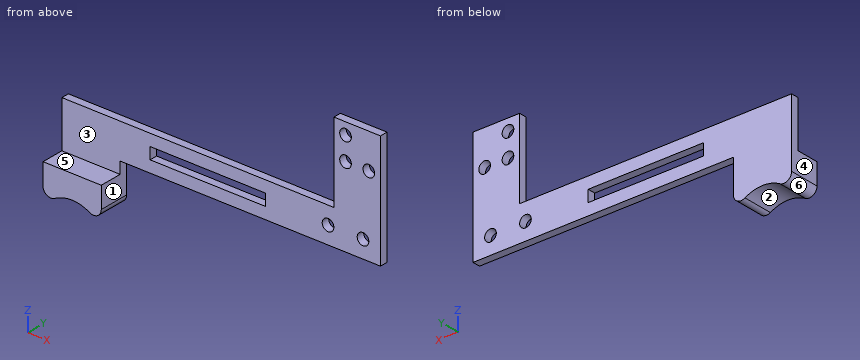
from build123d import *

# Parameters (mm, degrees)
F0_W      = 12
F0_H      = 16.5
F0_R      = 1.5
F0_W_2    = 15
F0_H_2    = 3
F1_DEPTH  = 2
F2_W      = 15
F2_H      = 7.8090135939
F3_DEPTH  = 10
F5_DEPTH  = 25
F6_R      = 2
F7_W      = 29.6666743584
F7_H      = 3
F8_DEPTH  = 25
F9_R      = 1.5
F10_DEPTH = 25


with BuildPart() as f1:
    # F0 (on Front) → F1 (new body)
    with BuildSketch(Plane.XZ):
        with Locations((3, -5.25)):
            Rectangle(F0_W, F0_H)
        with Locations((0, -6)):
            Circle(F0_R, mode=Mode.SUBTRACT)
        with Locations((6, -6)):
            Circle(F0_R, mode=Mode.SUBTRACT)
        Circle(F0_R, mode=Mode.SUBTRACT)
        Polygon((9, -13.5), (-3, -13.5), (-3, -17.375), (-3, -26.375), (9, -26.375), align=None)
        Polygon((-3, -26.375), (-3, -17.375), (-73, -17.375), (-73, -26.375), (-58, -26.375), align=None)
        with Locations((-65.5, -27.875)):
            Rectangle(F0_W_2, F0_H_2)
    extrude(amount=F1_DEPTH)

    # F2 (on face) → F3 (join)
    with BuildSketch(Plane(origin=(0, 0, -29.375), x_dir=(1, 0, 0), z_dir=(0, 0, -1))):
        with Locations((-65.5, 3.904506797)):
            Rectangle(F2_W, F2_H)
    extrude(amount=F3_DEPTH)

    # F4 (on face) → F5 (cut)
    with BuildSketch(Plane.XZ.offset(7.8090135939)):
        with BuildLine():
            Line((-73, -39.375), (-58, -39.375))
            ThreePointArc((-58, -39.375), (-65.5, -35.3883488839), (-73, -39.375))
        make_face()
    extrude(amount=-F5_DEPTH, mode=Mode.SUBTRACT)

    # F6
    f6_edges = [f1.edges().sort_by_distance(p)[0] for p in [
        (-73, -3.904507, -39.375),
        (-58, -3.904507, -39.375),
    ]]
    fillet(f6_edges, radius=F6_R)

    # F7 (on face) → F8 (cut)
    with BuildSketch(Plane.XZ.offset(2)):
        with Locations((-35.4711478576, -21.875)):
            Rectangle(F7_W, F7_H)
    extrude(amount=-F8_DEPTH, mode=Mode.SUBTRACT)

    # F9 (on face) → F10 (cut)
    with BuildSketch(Plane.XZ.offset(2)):
        with Locations((-4.5, -21.875)):
            Circle(F9_R)
        with Locations((4.5, -21.875)):
            Circle(F9_R)
    extrude(amount=-F10_DEPTH, mode=Mode.SUBTRACT)


solid = f1.part
Work out the finished part from the listing and answer in its coordinate system (mm). Face numbers are marked on the shaded views. A direction names the side the tool comes from. Round coordinates to 2 decimals unless told otherwise and drop trailing zeros. Write each loop counter-clockwise with the first axis right and the second up, starting at its lowest first coordinate (ties: lowest second). Pieces come first, ordered by that corner, then holes. Notation, with made-up numbers: M -10.75,62.25 L 40.25,62.25 A26 cw 40.25,91.25 Z; hole C 57.5,49.25 d6. An arc over 180 degrees is marked long. Use a Markdown table: item, result.
1) Determine the mould class of the marked faces 1, 2, 3 and 4 for opening direction X: pulls with the +X half, pulls with the -X half, needs draft (parallel to the pull), parting line crosses it, or undercut.
Taken from the geometry:
| item | result |
|---|---|
| face 1 | pulls with the +X half |
| face 2 | undercut |
| face 3 | needs draft |
| face 4 | pulls with the -X half |
2) Flat-ended cylindrical pins translate along their axes: pin 1 (1.6 mm diameter, centred on x = -35, y = -1.5, fed in from +Z) (3 decimals); pin 2 (3.5 mm diameter, centred on x = 4.5, z = -21.875, fed in from -Y); pin 3 (0.6 mm diameter, centred on y = -1, z = -8, fed in from -X); pin 4 (10 mm diameter, centred on x = -2, z = -28.5, fed in from +Y). Find the tip coordinate at first contact, or state that the pin passes through.
Taken from the geometry:
| item | result |
|---|---|
| pin 1 | stops at z = -17.375 |
| pin 2 | stops at y = -2 |
| pin 3 | stops at x = -3 |
| pin 4 | stops at y = 0 |
3) The part is cut by section C-C on z = 0. Give the vertices of the cut face in (x, y).
Taken from the geometry:
| item | result |
|---|---|
| outline | M -3,-2 L -1.5,-2 L -1.5,0 L -3,0 Z; M 1.5,-2 L 9,-2 L 9,0 L 1.5,0 Z |
4) Consider line 1 (Z direction, x = 0, y = -0.85) (3 decimals); line 2 (Z direction, x = -28, y = -1.25) (3 decimals); line 3 (X direction, y = -4.25, z = -31.5). Determine where each line is inside the solid, lowest interval first. Write a range as [from, to].
Taken from the geometry:
| item | result |
|---|---|
| line 1 | z = [-26.375, -7.5], [-4.5, -1.5], [1.5, 3] |
| line 2 | z = [-26.375, -23.375], [-20.375, -17.375] |
| line 3 | x = [-73, -58] |
5) Which of the six approach directions +Z, -Z, +X, -X, +Y, -Y give full straight-line access (tool end or side, diameter ignored) to the marked faces 5 and 6?
Taken from the geometry:
| item | result |
|---|---|
| face 5 | +Z, +X, -X, -Y |
| face 6 | -Z, +Y, -Y |
6) The part is cut by section B-B on x = 0. Give the vertices of the cut face in (y, z) (3 decimals).
Taken from the geometry:
| item | result |
|---|---|
| outline | M -2,-26.375 L 0,-26.375 L 0,-7.5 L -2,-7.5 Z; M -2,-4.5 L 0,-4.5 L 0,-1.5 L -2,-1.5 Z; M -2,1.5 L 0,1.5 L 0,3 L -2,3 Z |
7) The part is cut by section A-A on z = -6. Give the vertices of the cut face in (x, y).
Taken from the geometry:
| item | result |
|---|---|
| outline | M -3,-2 L -1.5,-2 L -1.5,0 L -3,0 Z; M 1.5,-2 L 4.5,-2 L 4.5,0 L 1.5,0 Z; M 7.5,-2 L 9,-2 L 9,0 L 7.5,0 Z |
8) The part is cut by section D-D on y = -0.75. Give the vertices of the cut face in (x, z) (3 decimals), plus the area to 3 significant figures.
Taken from the geometry:
| item | result |
|---|---|
| outline | M -73,-34.855 A2 ccw -70.004,-36.589 A9.048 cw -60.996,-36.589 A2 ccw -58,-34.855 L -58,-26.375 L 9,-26.375 L 9,3 L -3,3 L -3,-17.375 L -73,-17.375 Z; hole M -50.304,-23.375 L -20.638,-23.375 L -20.638,-20.375 L -50.304,-20.375 Z; hole C -4.5,-21.875 d3; hole C 0,-6 d3; hole C 0,0 d3; hole C 4.5,-21.875 d3; hole C 6,-6 d3 |
| area | 1,000 mm2 |
